Model file for the job. Use its own axes, mm. A direction names the side the tool comes from. Give positions to 0.01 mm unless a question says otherwise; leave off trailing zeros. Order: outer loops, then holes, each group sorted by start corner. A loop starts at its lowest first (then second) coordinate and runs counter-clockwise, first axis right, second up. Notation, with made-up numbers: (-16, 73) -> (22, 73) arc R8 cw to (22, 82) -> close; hole circle Ø3 at (67.25, -22). An arc over 180 degrees is marked (long way). Use CSV: the item, a comma, the result in double quotes. Start each with the question number.
1. Drop flat-ended pins along their axis: pin 1 (10.5 mm diameter, centred on x = 114, y = -17.5, fed in from +Z); pin 2 (13.5 mm diameter, centred on x = 74, z = 44.5, fed in from -Y); pin 3 (10.5 mm diameter, centred on y = -75.5, z = 41, fed in from +X). Give the stop position or say it passes through.
2. 3-axis set-ups, long thin cutter, end or side, ignore diameter. For faces 1 (the cylindrical face through (-24.92, -13.63, 101.24)), 2 (the flat face through (72, -30.419, 40)), 3 (the cylindrical face through (-1.61, -107.38, 51.45)): which of +Z, -Z, +X, -X, +Y, -Y reach the whole face in a straight line?
3. Cut at A-A on x = 0. List the corners of the cut face in (y, z), then the cut area to 3 significant figures.
4. Cut at C-C on y = -56. List the corners of the cut face in (x, z), then the cut area to 3 significant figures.
5. Cut at D-D on x = 109.5. List the corners of the cut face in (y, z), then the cut area to 3 significant figures.
6. Wall check: line 1 (Y direction, x = 29.5, z = 31); line 2 (Y direction, x = 78, z = 34.5); line 3 (X direction, y = -94, z = 27). Give the ranges that are in metal, low to high. Write a range as from..to.
7. Cut at B-B on z = 16.5. List the corners of the cut face in (x, y).
```python
from build123d import *

# Parameters (mm, degrees)
F0_W      = 101.6
F0_H      = 50.8
F0_R      = 16.775178
F1_DEPTH  = 50.8
F2_R      = 1.27
F2_R_2    = 12.7
F1_FACE_W = 101.6
F1_FACE_H = 50.8
F3_DEPTH  = 25.4
F4_R      = 12.7
F5_DEPTH  = 50.8
F6_W      = 24.609506
F6_H      = 44.177586
F7_DEPTH  = 50.8
F9_DEPTH  = 25.4
F11_DEPTH = 50.8
F12_R     = 12.394387
F13_DEPTH = 25.4


with BuildPart() as f1:
    # F0 (on Top) → F1 (new body)
    with BuildSketch(Plane.XY):
        with Locations((-3.902643, -18.653006)):
            Rectangle(F0_W, F0_H)
        with Locations((-16.602643, -18.653006)):
            Circle(F0_R, mode=Mode.SUBTRACT)
        with Locations((-16.602643, -18.653006)):
            Circle(F0_R)
    extrude(amount=F1_DEPTH)

    # F2 (on Top) + F1_face (on face) → F3 (join)
    with BuildSketch(Plane.XY):
        with Locations((-54.476865, -17.57852)):
            Circle(F2_R)
        with Locations((-32.452784, -17.5102)):
            Circle(F2_R_2)
    with BuildSketch(Plane(origin=(-3.902643, -18.653006, 50.8), x_dir=(1, 0, 0), z_dir=(0, 0, 1))):
        Rectangle(F1_FACE_W, F1_FACE_H)
    extrude(amount=F3_DEPTH)

    # F4 (on face) → F5 (join)
    with BuildSketch(Plane.XY.offset(76.2)):
        with Locations((-37.034646, -17.442938)):
            Circle(F4_R)
    extrude(amount=F5_DEPTH)

    # F6 (on face) → F7 (join)
    with BuildSketch(Plane.YZ.offset(46.897357)):
        with Locations((-18.113753, 40.772016)):
            Rectangle(F6_W, F6_H)
    extrude(amount=F7_DEPTH)

    # F8 (on face) → F9 (join)
    with BuildSketch(Plane.YZ.offset(97.697357)):
        Polygon((-22.591917, 42.024732), (-13.205347, 42.024732), (-8.512062, 50.15374), (-13.205347, 58.282748), (-22.591917, 58.282748), (-27.285202, 50.15374), align=None)
    extrude(amount=F9_DEPTH)

    # F10 (on face) → F11 (join)
    with BuildSketch(Plane.XZ.offset(44.053006)):
        Polygon((24.291333, 56.072608), (-26.942033, 56.072608), (-26.942033, 20.681137), (9.460622, 20.681137), (24.291333, 20.681137), (24.291333, 32.478295), align=None)
    extrude(amount=F11_DEPTH)

    # F12 (on face) → F13 (join)
    with BuildSketch(Plane.XZ.offset(94.853006)):
        with Locations((0, 39.159566)):
            Circle(F12_R)
    extrude(amount=F13_DEPTH)


solid = f1.part
```
Verdict:
1,pin 1,"z = 58.28"
1,pin 2,"y = -30.42"
1,pin 3,"x = 24.29"
2,face 1,"+Z"
2,face 2,"+Z, -Z, +X, -Y"
2,face 3,"-Y"
3,outline,"(-120.25, 26.77) -> (-94.85, 26.77) -> (-94.85, 20.68) -> (-44.05, 20.68) -> (-44.05, 0) -> (6.75, 0) -> (6.75, 76.2) -> (-44.05, 76.2) -> (-44.05, 56.07) -> (-94.85, 56.07) -> (-94.85, 51.55) -> (-120.25, 51.55) -> close"
3,area,"6,300 mm^2"
4,outline,"(-26.94, 20.68) -> (24.29, 20.68) -> (24.29, 56.07) -> (-26.94, 56.07) -> close"
4,area,"1,810 mm^2"
5,outline,"(-27.29, 50.15) -> (-22.59, 42.02) -> (-13.21, 42.02) -> (-8.51, 50.15) -> (-13.21, 58.28) -> (-22.59, 58.28) -> close"
5,area,"229 mm^2"
6,line 1,"-44.05..6.75"
6,line 2,"-30.42..-5.81"
6,line 3,"-26.94..24.29"
7,outline,"(-54.7, -44.05) -> (46.9, -44.05) -> (46.9, 6.75) -> (-54.7, 6.75) -> (-54.7, -16.33) arc R1.27 ccw to (-54.7, -18.83) -> close"
